Job drawing, mm, ordinate dimensions from the low corner. One solid piece. A direction names the side the tool comes from. Coordinates: 2 decimals unless noted, no trailing zeros. Order: outer loops, then holes, each group sorted by start corner. A loop starts at its lowest first (then second) coordinate and runs counter-clockwise, first axis right, second up. Notation, with made-up numbers: M 86,14.25 L 107,14.25 A8 ccw 107,18.25 Z; hole C 27.5,23.5 d11. An arc over 180 degrees is marked long. Write item = value, one per line.
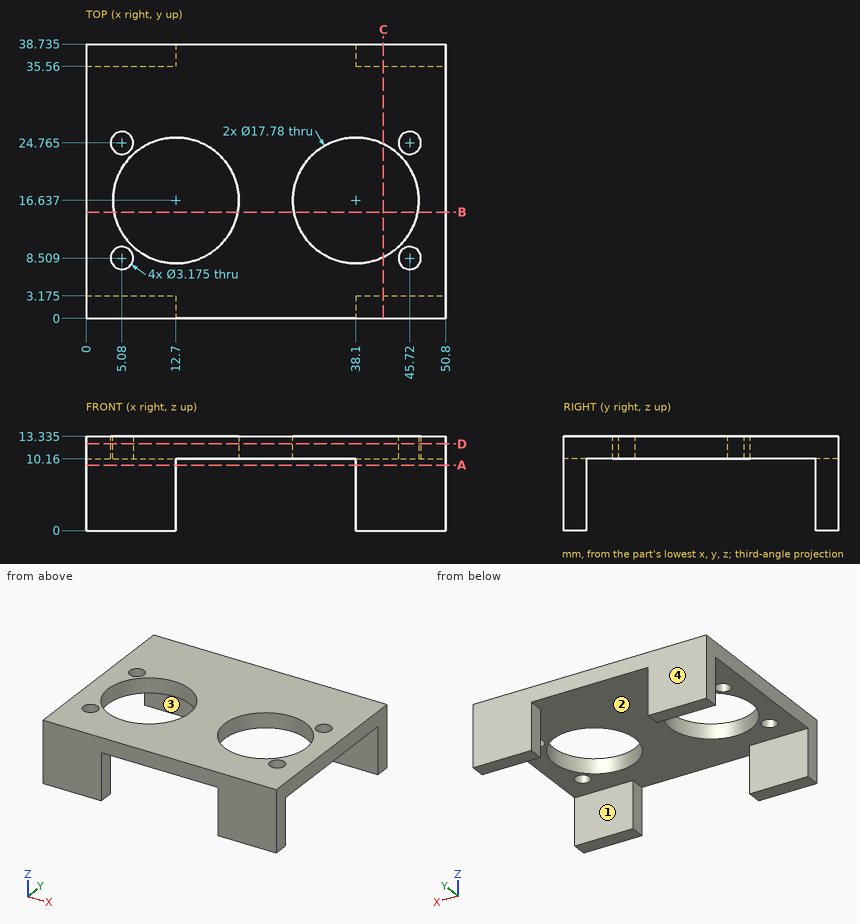
(1) Tool access for the marked faces 3 and 4: list every direction of +Z, -Z, +X, -X, +Y, -Y with a clear straight run to the whole face (end or side of a thin tool).
Evaluation:
face_3 = -Z, +X, -X
face_4 = +Z, -Z, +X, -X, +Y
(2) Slice it at D-D, the plane z = 12.25. Write the cut outline in (x, y) (1 decimal).
Evaluation:
outline = M 0,0 L 50.8,0 L 50.8,38.7 L 0,38.7 Z; hole C 5.1,8.5 d3.2; hole C 5.1,24.8 d3.2; hole C 12.7,16.6 d17.8; hole C 38.1,16.6 d17.8; hole C 45.7,8.5 d3.2; hole C 45.7,24.8 d3.2
(3) Pull direction X, two halves, no side cores. Call the marked faces 1 and 2: +X half, -X half, draft (parallel to the pull), parting line (faces both ways), or undercut.
Evaluation:
face_1 = draft
face_2 = undercut
(4) Slice it at C-C, the plane x = 42. Write the cut outline in (y, z) (3 decimals).
Evaluation:
outline = M 0,0 L 3.175,0 L 3.175,10.16 L 8.648,10.16 L 8.648,13.335 L 0,13.335 Z; M 24.626,10.16 L 35.56,10.16 L 35.56,0 L 38.735,0 L 38.735,13.335 L 24.626,13.335 Z
(5) Wall check: line 1 (X direction, y = 3, z = 10); line 2 (X direction, y = 19.5, z = 10.5); line 3 (Y direction, x = 38.5, z = 10.25) (3 decimals). Give the ranges that are in metal, low to high. Write a range as from..to.
Evaluation:
line_1 = 0..12.7, 38.1..50.8
line_2 = 0..4.28, 21.12..29.68, 46.52..50.8
line_3 = 0..7.756, 25.518..38.735
(6) Slice it at B-B, the plane y = 15. Write the cut outline in (x, z) (3 decimals).
Evaluation:
outline = M 0,10.16 L 3.962,10.16 L 3.962,13.335 L 0,13.335 Z; M 21.438,10.16 L 29.362,10.16 L 29.362,13.335 L 21.438,13.335 Z; M 46.838,10.16 L 50.8,10.16 L 50.8,13.335 L 46.838,13.335 Z
(7) Pin check, flat tips, straight feed: pin 1 Ø3.5 at (x, y) = (45.72, 8.509) entering from -Z; pin 2 Ø1.9 at (x, y) = (5.08, 8.509) entering from -Z. Stop position of each tip, or through.
Evaluation:
pin_1 = 10.16
pin_2 = through
(8) Slice it at A-A, the plane z = 9.25. Write the cut outline in (x, y) (3 decimals).
Evaluation:
outline = M 0,0 L 12.7,0 L 12.7,3.175 L 0,3.175 Z; M 0,35.56 L 12.7,35.56 L 12.7,38.735 L 0,38.735 Z; M 38.1,0 L 50.8,0 L 50.8,3.175 L 38.1,3.175 Z; M 38.1,35.56 L 50.8,35.56 L 50.8,38.735 L 38.1,38.735 Z
